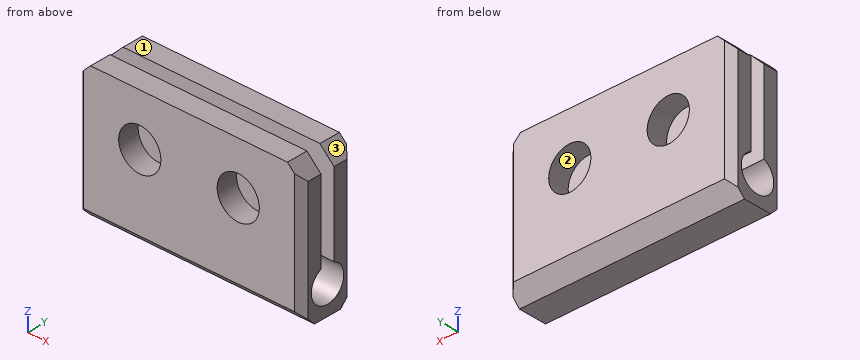
Autodesk Inventor part; units mm, degrees
ref_plane "YZ Plane" through (0, 0, 0) normal (1, 0, 0) x (0, 1, 0)
ref_plane "XZ Plane" through (0, 0, 0) normal (0, 1, 0) x (-1, 0, 0)
ref_plane "XY Plane" through (0, 0, 0) normal (0, 0, 1) x (1, 0, 0)
sketch "Esboço1" plane through (0, 0, 0) normal (0, 1, 0) x (-1, 0, 0)
  line L0 (-8, -5) -> (8, -5)
  line L1 (8, -5) -> (8, 5)
  line L2 (8, 5) -> (-8, 5)
  line L3 (-8, 5) -> (-8, -5)
  line L4 (-8, -5) -> (8, 5) construction
  line L5 (8, -5) -> (-8, 5) construction
  point P0 (0, 0)
  dimension "d0" = 16
  dimension "d1" = 10
extrude "Extrusão1" add sketch "Esboço1" along normal blind 4
sketch "Esboço2" plane through (8, 0, 5) normal (1, 0, 0) x (0, 0, -1)
  line L0 (0, 0) -> (0, 4)
  line L1 (10, 0) -> (10, 4)
  arc A0 (6.8544, 1.5) -> (6.8544, 2.5) centre (8, 2) ccw
  line L2 (-0.795, 1.5) -> (-0.795, 2.5)
  line L3 (-0.795, 2.5) -> (6.8544, 2.5)
  line L4 (6.8544, 1.5) -> (-0.795, 1.5)
  point P0 (5, 0)
  point P1 (0, 2.5)
  point P2 (0, 1.5)
  dimension "d7" = 2.5
  dimension "d8" = 1
extrude "Extrusão2" cut sketch "Esboço2" against normal through all contours L0 L3 A0 L4
chamfer "Chanfro1" distance 1 angle 45 4 edges at (-8, 3.25, 5) (-8, 0.75, 5) (8, 0.75, 5) (8, 3.25, 5)
chamfer "Chanfro2" distance 1 angle 45 2 edges at (0, 4, -5) (0, 0, -5)
chamfer "Chanfro3" distance 0.5 angle 45 4 edges at (8, 4, 0) (8, 0, 0) (-8, 4, 0) (-8, 0, 0)
sketch "Esboço3" plane through (0, 4, 0) normal (0, 1, 0) x (1, 0, 0)
  line L0 (-7.5, -4.5) -> (-7.5, 4)
  line L1 (7, -5) -> (8, -4)
  line L2 (-7.5, 4) -> (7.5, 4)
  line L3 (7.5, 4) -> (7.5, -4.5)
  line L4 (7.5, -4.5) -> (-7.5, -4.5)
  line L5 (-7.5, -4.5) -> (-7.5, 4)
  line L6 (8, 1.8544) -> (-8, 1.8544)
  line L7 (-7.5, 1.8544) -> (7.5, 1.8544)
  line L8 (7.5, 1.8544) -> (7.5, -4.5)
  line L9 (7.5, -4.5) -> (-7.5, -4.5)
  line L10 (-7.5, -4.5) -> (-7.5, 1.8544)
  line L11 (-7.5, -1.3228) -> (7.5, -1.3228)
  line L12 (-7.5, -1.3228) -> (-3.5, -1.3228)
  circle A0 centre (-3.5, -1.3228) radius 1.5
  line L13 (7.5, -1.3228) -> (3.5, -1.3228)
  circle A1 centre (3.5, -1.3228) radius 1.5
  point P0 (0, 0)
  dimension "d20" = 4
  dimension "d21" = 3
  dimension "d22" = 4
  dimension "d23" = 3
extrude "Extrusão3" cut sketch "Esboço3" against normal through all contours A0 L11 | L11 A0 | A1 L11 | L11 A1
properties part number "Sup_haste_corpo"
Source: CAD feature listing. Evaluate the final solid. Frame: model axes, mm. Face numbers are marked on the shaded views. Coordinates: 2 decimals unless noted, no trailing zeros. Loops run counter-clockwise (first coordinate to the right, second up) from the corner with the lowest first, then second, coordinate; pieces in that order, holes last. Notation, with made-up numbers: (63, 5.25) -> (83, 5.25) arc R13 ccw to (83, 13.25) -> close; hole circle Ø1 at (25, 73). An arc over 180 degrees is marked (long way). One line per item, written item: value. Start each with the question number.
Q1. Line query: line 1 along Y through (x, z) = (3, -0.5); line 2 along Y through (x, z) = (-5, -2.25); line 3 along X through (y, z) = (2.65, 2). Output: solid intervals per line, ascending.
Q2. Section query C-C, the plane z = 2.5. Return the cut outline in (x, y), and give its area (3 significant figures).
Q3. Section query D-D, the plane y = 2. Return the cut outline in (x, z), and give its area (3 significant figures).
Q4. Section query B-B, the plane z = -3. Return the cut outline in (x, y).
Q5. Mould query, pull axis X, two halves, no side actions, for the marked faces 1, 2 and 3. Classes: pulls with the +X half, pulls with the -X half, needs draft (parallel to the pull), parting line crosses it, or undercut.
Q6. Section query A-A, the plane x = 3.5. Return the cut outline in (y, z), and give its area (3 significant figures).
Results:
1. line 1: 0 to 1.5, 2.5 to 4
1. line 2: 0 to 1, 3 to 4
1. line 3: -8 to -4.84, -2.16 to 2.16, 4.84 to 8
2. outline: (-8, 0.5) -> (-7.5, 0) -> (-4.43, 0) -> (-4.43, 1.5) -> (-8, 1.5) -> close; (-8, 2.5) -> (-4.43, 2.5) -> (-4.43, 4) -> (-7.5, 4) -> (-8, 3.5) -> close; (-2.57, 0) -> (2.57, 0) -> (2.57, 1.5) -> (-2.57, 1.5) -> close; (-2.57, 2.5) -> (2.57, 2.5) -> (2.57, 4) -> (-2.57, 4) -> close; (4.43, 0) -> (7.5, 0) -> (8, 0.5) -> (8, 1.5) -> (4.43, 1.5) -> close; (4.43, 2.5) -> (8, 2.5) -> (8, 3.5) -> (7.5, 4) -> (4.43, 4) -> close
2. area: 36.3 mm^2
3. outline: (-8, -5) -> (8, -5) -> (8, -4.25) -> (-8, -4.25) -> close
3. area: 12.0 mm^2
4. outline: (-8, 0.5) -> (-7.5, 0) -> (7.5, 0) -> (8, 0.5) -> (8, 0.75) -> (-8, 0.75) -> close; (-8, 3.25) -> (8, 3.25) -> (8, 3.5) -> (7.5, 4) -> (-7.5, 4) -> (-8, 3.5) -> close
5. face 1: needs draft
5. face 2: undercut
5. face 3: pulls with the +X half
6. outline: (0, -4) -> (1, -5) -> (3, -5) -> (4, -4) -> (4, -0.18) -> (2.5, -0.18) -> (2.5, -1.85) arc R1.25 cw (long way) to (1.5, -1.85) -> (1.5, -0.18) -> (0, -0.18) -> close; (0, 2.82) -> (1.5, 2.82) -> (1.5, 5) -> (0, 5) -> close; (2.5, 2.82) -> (4, 2.82) -> (4, 5) -> (2.5, 5) -> close
6. area: 18.3 mm^2
